from build123d import *

# Parameters (mm, degrees)
F0_W        = 36
F0_H        = 67.1
F1_DEPTH    = 7.3
F2_R        = 4.2454518292
F3_DEPTH    = 0.4
F5_SIZE     = 2
F6_T1_DEPTH = 81.5974746831
F4_W        = 30
F4_H        = 50
F7_DEPTH    = 1
F8_T1_DEPTH = 102.1


# Not quite as in the source:
# - a fillet or chamfer that OpenCascade refuses, or shapes differently, is made with other operations: its cross-section is extruded or revolved along the edge and cut away or added


with BuildPart() as f1:
    # F0 (on Top) → F1 (new body)
    with BuildSketch(Plane.XY):
        Rectangle(F0_W, F0_H)
    extrude(amount=F1_DEPTH)

    # F2 (on face) → F3 (cut)
    with BuildSketch(Plane.XY.offset(7.3)):
        with Locations((0, -26.7354752868)):
            Circle(F2_R)
    extrude(amount=-F3_DEPTH, mode=Mode.SUBTRACT)

    # F5
    f5_edges = [f1.edges().sort_by_distance(p)[0] for p in [
        (18, 0, 7.3),
    ]]
    chamfer(f5_edges, length=F5_SIZE)

    # F6: fillet of radius 7 on 1 edges, made by hand

    # F6_s2 → F6_t1 (cut)
    with BuildSketch(Plane.XZ.offset(-40.7987373415)):
        with BuildLine():
            ThreePointArc((18, 2.4005050634), (17.4671567276, 5.0792890899), (15.9497474683, 7.3502525317))
            Line((15.9497474683, 7.3502525317), (18, 5.3))
            Line((18, 5.3), (18, 2.4005050634))
        make_face()
    extrude(amount=F6_T1_DEPTH, mode=Mode.SUBTRACT)

    # F4 (on face) → F7 (cut)
    with BuildSketch(Plane.XY.offset(7.3)):
        with Locations((0, 4.2591368308)):
            Rectangle(F4_W, F4_H)
    extrude(amount=-F7_DEPTH, mode=Mode.SUBTRACT)

    # F8: fillet of radius 7 on 1 edges, made by hand

    # F8_s2 → F8_t1 (cut)
    with BuildSketch(Plane.XZ.offset(-51.05)):
        with BuildLine():
            ThreePointArc((-18, 0.3), (-15.9497474683, 5.2497474683), (-11, 7.3))
            Line((-11, 7.3), (-18, 7.3))
            Line((-18, 7.3), (-18, 0.3))
        make_face()
    extrude(amount=F8_T1_DEPTH, mode=Mode.SUBTRACT)


solid = f1.part
Verification items for the finished model (mm, model axes). A direction names the side the tool comes from. Coordinates: 2 decimals unless noted, no trailing zeros. Write each loop counter-clockwise with the first axis right and the second up, starting at its lowest first coordinate (ties: lowest second). Pieces come first, ordered by that corner, then holes. Notation, with made-up numbers: M -6.75,81 L 15.25,81 A27 ccw 15.25,98 Z; hole C -14,71.25 d4. An arc over 180 degrees is marked long. Use a Markdown table: item, result.
Q1. Sectioned sample at D-D, the plane z = 3.5. Record the boundary of the cut face in (x, y), plus the area to 3 significant figures.
Reply:
| item | result |
|---|---|
| outline | M -17.23,-33.55 L 17.91,-33.55 L 17.91,33.55 L -17.23,33.55 Z |
| area | 2,360 mm² |
Q2. Thickness scan on line 1 (Y direction, x = 0, z = 7.2); line 2 (Z direction, x = 5, y = 13); line 3 (X direction, y = -27.5, z = 0.5). Record the ranges inside material, lowest first.
Reply:
| item | result |
|---|---|
| line 1 | y = -33.55 to -30.98, -22.49 to -20.74, 29.26 to 33.55 |
| line 2 | z = 0 to 6.3 |
| line 3 | x = -18 to 18 |
Q3. Sectioned sample at C-C, the plane x = -13. Record the boundary of the cut face in (y, z), plus the area to 3 significant figures.
Reply:
| item | result |
|---|---|
| outline | M -33.55,0 L 33.55,0 L 33.55,7.01 L 29.26,7.01 L 29.26,6.3 L -20.74,6.3 L -20.74,7.01 L -33.55,7.01 Z |
| area | 435 mm² |
Q4. Set-up check for faces 4 (the face through (17.5, 0.5, 5)), 5 (the face through (0, -27, 6.9)), 6 (the face through (0, 5, 6.3)): record each of +Z, -Z, +X, -X, +Y, -Y from which the full face is reachable in a straight line by a thin tool's end or side.
Reply:
| item | result |
|---|---|
| face 4 | +Z, +X, +Y, -Y |
| face 5 | +Z |
| face 6 | +Z, -X |
Q5. Sectioned sample at B-B, the plane x = 0. Record the boundary of the cut face in (y, z), plus the area to 3 significant figures.
Reply:
| item | result |
|---|---|
| outline | M -33.55,0 L 33.55,0 L 33.55,7.3 L 29.26,7.3 L 29.26,6.3 L -20.74,6.3 L -20.74,7.3 L -22.49,7.3 L -22.49,6.9 L -30.98,6.9 L -30.98,7.3 L -33.55,7.3 Z |
| area | 436 mm² |
Q6. Go/stop test with flat-tipped pins: P1, Ø2, axis at x = 1, y = 6.5, coming from the +Z side; P2, Ø5, axis at x = 0, y = -26.74, coming from the +Z side; P3, Ø1.5, axis at x = 12, y = 18.5, coming from the -Z side; P4, Ø4, axis at y = -2.5, z = 3.5, coming from the -X side. Record where each tip stops, or that it passes through.
Reply:
| item | result |
|---|---|
| P1 | stops at z = 6.3 |
| P2 | stops at z = 6.9 |
| P3 | stops at z = 0 |
| P4 | stops at x = -17.9 |
Q7. Sectioned sample at A-A, the plane y = 23.5. Record the boundary of the cut face in (x, z).
Reply:
| item | result |
|---|---|
| outline | M -18,0 L 18,0 L 18,2.4 A7 ccw 16,7.3 L 15,7.3 L 15,6.3 L -14.61,6.3 A7 ccw -18,0.3 Z |
Q8. Draft check along Y on faces 1 (the face through (-0.92, -30.88, 7.1)), 2 (the face through (18, 0, 1)), 3 (the face through (0, -33.55, 4)). Enter one of: +Y half, -Y half, draft (parallel to the pull), parting line (faces both ways), or undercut.
Reply:
| item | result |
|---|---|
| face 1 | undercut |
| face 2 | draft |
| face 3 | -Y half |
